Geometry: see drawing. Coordinates: mm, zero at the bounding-box minimum. A direction names the side the tool comes from. Give positions to 0.01 mm unless a question says otherwise; leave off trailing zeros. Write each loop counter-clockwise with the first axis right and the second up, starting at its lowest first coordinate (ties: lowest second). Pieces come first, ordered by that corner, then holes. Notation, with made-up numbers: M 65.5,-13 L 71.5,-13 A21 cw 71.5,7 Z; hole C -23.5,-21 d2. An arc over 180 degrees is marked long. Use CSV: the item, a comma, the result in double quotes. Start each with the question number.
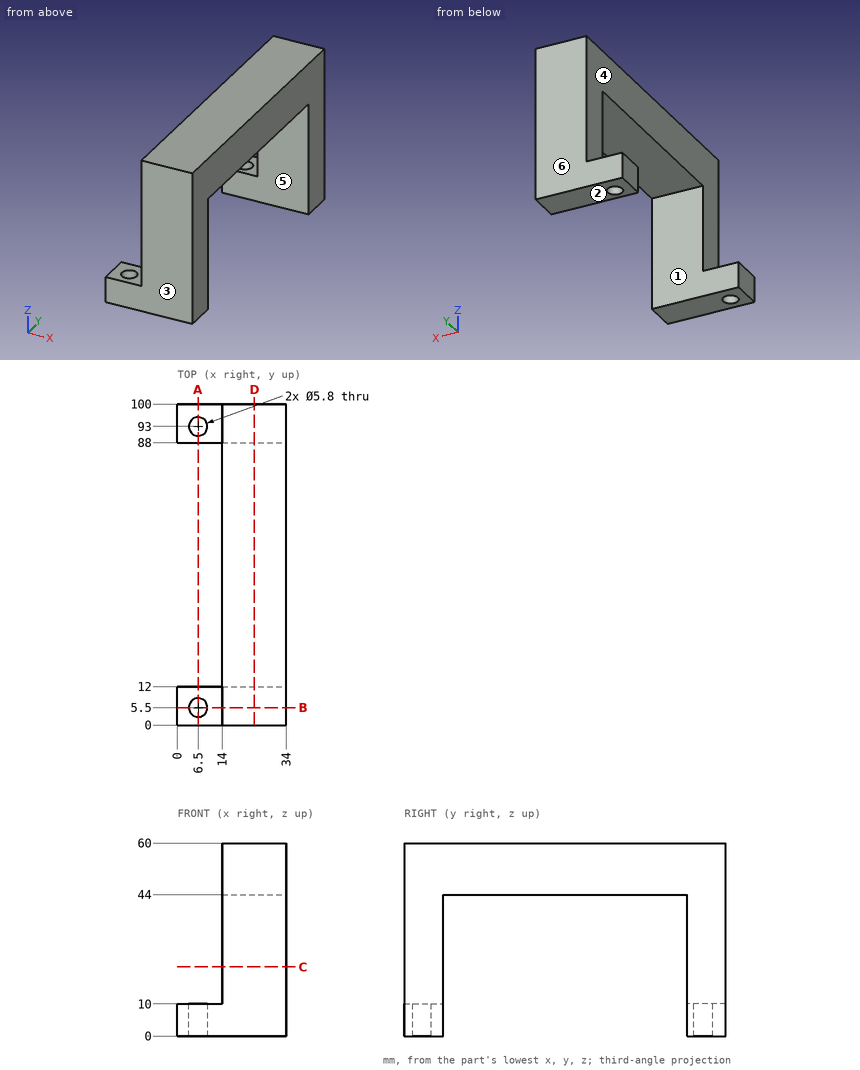
1. Line query: probe 1 along Y at (x, z) = (17, 8.5); probe 2 along X at (y, z) = (93, 5.75); probe 3 along Y at (x, z) = (6.5, 4.5). Output: solid intervals per line, ascending.
2. Section D-D on x = 24. Return loops of the section in (y, z).
3. First-contact query: pin 1 (6 mm diameter, centred on x = 22.5, y = 48, fed in from -Z); pin 2 (6 mm diameter, centred on x = 10.5, y = 5.5, fed in from +Z); pin 3 (4.5 mm diameter, centred on x = 6.5, y = 5.5, fed in from +Z). Flat tips, straight axial feed; report the tip coordinate or a pass-through.
4. Section B-B on y = 5.5. Return loops of the section in (x, z).
5. Section C-C on z = 21.5. Return loops of the section in (x, y), then the cut area to 3 significant figures.
6. Pull-direction query (Y, two-part tool) for the marked faces 1, 2 and 3; classes: released by +Y, released by -Y, zero draft, split by the parting line, or undercut.
7. Access query for the marked faces 4, 5 and 6. Directions: +Z, -Z, +X, -X, +Y, -Y. A direction counts if a zero-diameter tool reaches every point of the face in a straight line with its end or side. Return the directions, or none.
8. Section A-A on x = 6.5. Return loops of the section in (y, z).
Resolved:
1,probe 1,"y = 0 to 12, 88 to 100"
1,probe 2,"x = 0 to 3.6, 9.4 to 34"
1,probe 3,"y = 0 to 2.6, 8.4 to 12, 88 to 90.1, 95.9 to 100"
2,outline,"M 0,0 L 12,0 L 12,44 L 88,44 L 88,0 L 100,0 L 100,60 L 0,60 Z"
3,pin 1,"stops at z = 44"
3,pin 2,"stops at z = 10"
3,pin 3,"passes through"
4,outline,"M 0,0 L 3.6,0 L 3.6,10 L 0,10 Z; M 9.4,0 L 34,0 L 34,60 L 14,60 L 14,10 L 9.4,10 Z"
5,outline,"M 14,0 L 34,0 L 34,12 L 14,12 Z; M 14,88 L 34,88 L 34,100 L 14,100 Z"
5,area,"480 mm2"
6,face 1,"undercut"
6,face 2,"zero draft"
6,face 3,"released by -Y"
7,face 4,"+Z, -X, +Y, -Y"
7,face 5,"-Z, +X, -X"
7,face 6,"+Z, -Z, +X, -X, +Y"
8,outline,"M 0,0 L 2.6,0 L 2.6,10 L 0,10 Z; M 8.4,0 L 12,0 L 12,10 L 8.4,10 Z; M 88,0 L 90.1,0 L 90.1,10 L 88,10 Z; M 95.9,0 L 100,0 L 100,10 L 95.9,10 Z"
